Read the model definition and answer for the solid it produces. Units are mm, in the model's axes. Face numbers are marked on the shaded views. A direction names the side the tool comes from. Coordinates: 2 decimals unless noted, no trailing zeros. Write each loop counter-clockwise with the first axis right and the second up, starting at its lowest first coordinate (ties: lowest second). Pieces come first, ordered by that corner, then holes.
1) Find the intervals of material crossed by line 1 (Z direction, x = 0.75, y = -3); line 2 (Y direction, x = -0.25, z = 3); line 3 (X direction, y = -0.25, z = 36), in increasing order.
2) The part is cut by section D-D (x = -3.5). Determine the outline of the cut face in (y, z), then the cut area to 3 significant figures.
3) Each of these flat-tipped pins is pushed along its axis until it touches: pin 1 Ø2.5 at (x, y) = (1.5, -2) entering from -Z; pin 2 Ø3 at (x, y) = (3, -3) entering from -Z; pin 3 Ø1.5 at (x, z) = (-1, 45.5) entering from -Y. Where does it stop, or does it pass through?
4) The part is cut by section C-C (z = 27.5). Determine the outline of the cut face in (x, y).
5) Which of the six approach directions +Z, -Z, +X, -X, +Y, -Y give full straight-line access (tool end or side, diameter ignored) to the marked faces 1 and 2?
6) The part is cut by section A-A (x = 0). Determine the outline of the cut face in (y, z).
from build123d import *

# Parameters (mm, degrees)
ESQUISSE1_R        = 3
BOSS_EXTRU_1_DEPTH = 8
CHANFREIN1_SIZE    = 0.5
ESQUISSE2_R        = 4
BOSS_EXTRU_2_DEPTH = 50


with BuildPart() as part:
    # Esquisse1 → Boss.-Extru.1 (new body)
    with BuildSketch(Plane.XY):
        Circle(ESQUISSE1_R)
    extrude(amount=BOSS_EXTRU_1_DEPTH)

    # Chanfrein1
    chanfrein1_edges = [part.edges().sort_by_distance(p)[0] for p in [
        (-3, 0, 0),
    ]]
    chamfer(chanfrein1_edges, length=CHANFREIN1_SIZE)

    # Esquisse2 → Boss.-Extru.2 (add)
    with BuildSketch(Plane.XY.offset(8)):
        Circle(ESQUISSE2_R)
    extrude(amount=BOSS_EXTRU_2_DEPTH)


solid = part.part
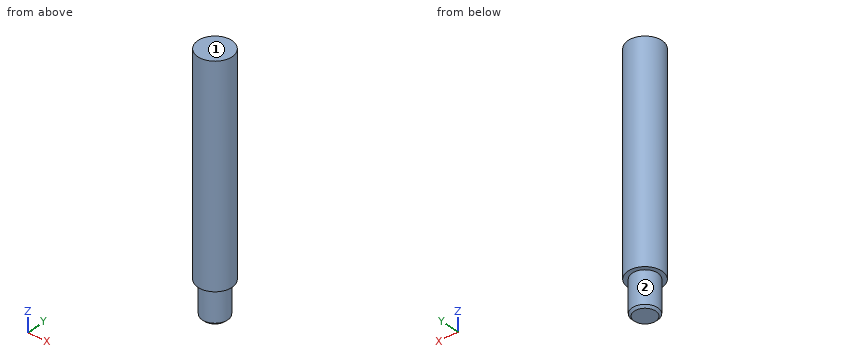
Reported:
1. line 1: z = 8 to 58
1. line 2: y = -2.99 to 2.99
1. line 3: x = -3.99 to 3.99
2. outline: (-1.94, 8) - (1.94, 8) - (1.94, 58) - (-1.94, 58) - close
2. area: 194 mm2
3. pin 1: stops at z = 0
3. pin 2: stops at z = 0.24
3. pin 3: stops at y = -3.99
4. outline: circle Ø8 at (0, 0)
5. face 1: +Z, +X, -X, +Y, -Y
5. face 2: -Z
6. outline: (-4, 8) - (-3, 8) - (-3, 0.5) - (-2.5, 0) - (2.5, 0) - (3, 0.5) - (3, 8) - (4, 8) - (4, 58) - (-4, 58) - close
